from build123d import *

# Parameters (mm, degrees)
F0_R     = 2.4
F1_DEPTH = 3.7
F0_R_2   = 40
F2_DEPTH = 2
F3_R     = 0.5


with BuildPart() as f1:
    # F0 (on Top) → F1 (new body)
    with BuildSketch(Plane.XY):
        with Locations((8, 16)):
            Circle(F0_R)
        with Locations((16, 8)):
            Circle(F0_R)
        with Locations((24, 8)):
            Circle(F0_R)
        with Locations((16, 16)):
            Circle(F0_R)
        with Locations((24, 16)):
            Circle(F0_R)
        with Locations((32, 0)):
            Circle(F0_R)
        with Locations((32, 8)):
            Circle(F0_R)
        with Locations((32, 16)):
            Circle(F0_R)
        with Locations((32, 24)):
            Circle(F0_R)
        with Locations((24, 24)):
            Circle(F0_R)
        with Locations((16, 24)):
            Circle(F0_R)
        with Locations((8, 24)):
            Circle(F0_R)
        with Locations((0, 32)):
            Circle(F0_R)
        with Locations((8, 32)):
            Circle(F0_R)
        with Locations((16, 32)):
            Circle(F0_R)
        with Locations((24, 32)):
            Circle(F0_R)
        with Locations((32, 32)):
            Circle(F0_R)
        with Locations((32, 40)):
            Circle(F0_R)
        with Locations((24, 40)):
            Circle(F0_R)
        with Locations((16, 40)):
            Circle(F0_R)
        with Locations((8, 40)):
            Circle(F0_R)
        with Locations((0, 40)):
            Circle(F0_R)
        with Locations((8, 48)):
            Circle(F0_R)
        with Locations((16, 48)):
            Circle(F0_R)
        with Locations((32, 48)):
            Circle(F0_R)
        with Locations((32, 56)):
            Circle(F0_R)
        with Locations((24, 56)):
            Circle(F0_R)
        with Locations((16, 56)):
            Circle(F0_R)
        with Locations((8, 56)):
            Circle(F0_R)
        with Locations((24, 48)):
            Circle(F0_R)
        with Locations((16, 64)):
            Circle(F0_R)
        with Locations((24, 64)):
            Circle(F0_R)
        with Locations((32, 64)):
            Circle(F0_R)
        with Locations((32, 72)):
            Circle(F0_R)
        with Locations((40, 72)):
            Circle(F0_R)
        with Locations((40, 64)):
            Circle(F0_R)
        with Locations((40, 56)):
            Circle(F0_R)
        with Locations((40, 48)):
            Circle(F0_R)
        with Locations((40, 40)):
            Circle(F0_R)
        with Locations((40, 32)):
            Circle(F0_R)
        with Locations((40, 24)):
            Circle(F0_R)
        with Locations((40, 16)):
            Circle(F0_R)
        with Locations((40, 8)):
            Circle(F0_R)
        with Locations((40, 0)):
            Circle(F0_R)
        with Locations((48, 8)):
            Circle(F0_R)
        with Locations((48, 16)):
            Circle(F0_R)
        with Locations((48, 24)):
            Circle(F0_R)
        with Locations((48, 32)):
            Circle(F0_R)
        with Locations((48, 40)):
            Circle(F0_R)
        with Locations((48, 48)):
            Circle(F0_R)
        with Locations((48, 56)):
            Circle(F0_R)
        with Locations((48, 64)):
            Circle(F0_R)
        with Locations((56, 64)):
            Circle(F0_R)
        with Locations((56, 56)):
            Circle(F0_R)
        with Locations((56, 48)):
            Circle(F0_R)
        with Locations((56, 40)):
            Circle(F0_R)
        with Locations((56, 32)):
            Circle(F0_R)
        with Locations((56, 24)):
            Circle(F0_R)
        with Locations((56, 16)):
            Circle(F0_R)
        with Locations((56, 8)):
            Circle(F0_R)
        with Locations((64, 16)):
            Circle(F0_R)
        with Locations((64, 24)):
            Circle(F0_R)
        with Locations((64, 32)):
            Circle(F0_R)
        with Locations((64, 40)):
            Circle(F0_R)
        with Locations((64, 48)):
            Circle(F0_R)
        with Locations((64, 56)):
            Circle(F0_R)
        with Locations((72, 40)):
            Circle(F0_R)
        with Locations((72, 32)):
            Circle(F0_R)
    extrude(amount=F1_DEPTH)

    # F0 (on Top) → F2 (join)
    with BuildSketch(Plane.XY):
        with Locations((36, 36)):
            Circle(F0_R_2)
        with Locations((32, 0)):
            Circle(F0_R, mode=Mode.SUBTRACT)
        with Locations((16, 8)):
            Circle(F0_R, mode=Mode.SUBTRACT)
        with Locations((24, 8)):
            Circle(F0_R, mode=Mode.SUBTRACT)
        with Locations((32, 8)):
            Circle(F0_R, mode=Mode.SUBTRACT)
        with Locations((8, 16)):
            Circle(F0_R, mode=Mode.SUBTRACT)
        with Locations((8, 24)):
            Circle(F0_R, mode=Mode.SUBTRACT)
        with Locations((0, 32)):
            Circle(F0_R, mode=Mode.SUBTRACT)
        with Locations((8, 32)):
            Circle(F0_R, mode=Mode.SUBTRACT)
        with Locations((16, 16)):
            Circle(F0_R, mode=Mode.SUBTRACT)
        with Locations((24, 16)):
            Circle(F0_R, mode=Mode.SUBTRACT)
        with Locations((16, 24)):
            Circle(F0_R, mode=Mode.SUBTRACT)
        with Locations((24, 24)):
            Circle(F0_R, mode=Mode.SUBTRACT)
        with Locations((32, 16)):
            Circle(F0_R, mode=Mode.SUBTRACT)
        with Locations((32, 24)):
            Circle(F0_R, mode=Mode.SUBTRACT)
        with Locations((16, 32)):
            Circle(F0_R, mode=Mode.SUBTRACT)
        with Locations((24, 32)):
            Circle(F0_R, mode=Mode.SUBTRACT)
        with Locations((32, 32)):
            Circle(F0_R, mode=Mode.SUBTRACT)
        with Locations((40, 0)):
            Circle(F0_R, mode=Mode.SUBTRACT)
        with Locations((40, 8)):
            Circle(F0_R, mode=Mode.SUBTRACT)
        with Locations((48, 8)):
            Circle(F0_R, mode=Mode.SUBTRACT)
        with Locations((56, 8)):
            Circle(F0_R, mode=Mode.SUBTRACT)
        with Locations((40, 16)):
            Circle(F0_R, mode=Mode.SUBTRACT)
        with Locations((40, 24)):
            Circle(F0_R, mode=Mode.SUBTRACT)
        with Locations((48, 16)):
            Circle(F0_R, mode=Mode.SUBTRACT)
        with Locations((48, 24)):
            Circle(F0_R, mode=Mode.SUBTRACT)
        with Locations((40, 32)):
            Circle(F0_R, mode=Mode.SUBTRACT)
        with Locations((48, 32)):
            Circle(F0_R, mode=Mode.SUBTRACT)
        with Locations((56, 16)):
            Circle(F0_R, mode=Mode.SUBTRACT)
        with Locations((64, 16)):
            Circle(F0_R, mode=Mode.SUBTRACT)
        with Locations((56, 24)):
            Circle(F0_R, mode=Mode.SUBTRACT)
        with Locations((64, 24)):
            Circle(F0_R, mode=Mode.SUBTRACT)
        with Locations((56, 32)):
            Circle(F0_R, mode=Mode.SUBTRACT)
        with Locations((64, 32)):
            Circle(F0_R, mode=Mode.SUBTRACT)
        with Locations((72, 32)):
            Circle(F0_R, mode=Mode.SUBTRACT)
        with Locations((0, 40)):
            Circle(F0_R, mode=Mode.SUBTRACT)
        with Locations((8, 40)):
            Circle(F0_R, mode=Mode.SUBTRACT)
        with Locations((8, 48)):
            Circle(F0_R, mode=Mode.SUBTRACT)
        with Locations((16, 40)):
            Circle(F0_R, mode=Mode.SUBTRACT)
        with Locations((24, 40)):
            Circle(F0_R, mode=Mode.SUBTRACT)
        with Locations((32, 40)):
            Circle(F0_R, mode=Mode.SUBTRACT)
        with Locations((16, 48)):
            Circle(F0_R, mode=Mode.SUBTRACT)
        with Locations((24, 48)):
            Circle(F0_R, mode=Mode.SUBTRACT)
        with Locations((32, 48)):
            Circle(F0_R, mode=Mode.SUBTRACT)
        with Locations((8, 56)):
            Circle(F0_R, mode=Mode.SUBTRACT)
        with Locations((16, 56)):
            Circle(F0_R, mode=Mode.SUBTRACT)
        with Locations((24, 56)):
            Circle(F0_R, mode=Mode.SUBTRACT)
        with Locations((16, 64)):
            Circle(F0_R, mode=Mode.SUBTRACT)
        with Locations((24, 64)):
            Circle(F0_R, mode=Mode.SUBTRACT)
        with Locations((32, 56)):
            Circle(F0_R, mode=Mode.SUBTRACT)
        with Locations((32, 64)):
            Circle(F0_R, mode=Mode.SUBTRACT)
        with Locations((32, 72)):
            Circle(F0_R, mode=Mode.SUBTRACT)
        Polygon((37, 33.5), (35, 33.5), (35, 35), (33.5, 35), (33.5, 37), (35, 37), (35, 38.5), (37, 38.5), (37, 37), (38.5, 37), (38.5, 35), (37, 35), align=None, mode=Mode.SUBTRACT)
        with Locations((40, 40)):
            Circle(F0_R, mode=Mode.SUBTRACT)
        with Locations((48, 40)):
            Circle(F0_R, mode=Mode.SUBTRACT)
        with Locations((40, 48)):
            Circle(F0_R, mode=Mode.SUBTRACT)
        with Locations((48, 48)):
            Circle(F0_R, mode=Mode.SUBTRACT)
        with Locations((56, 40)):
            Circle(F0_R, mode=Mode.SUBTRACT)
        with Locations((64, 40)):
            Circle(F0_R, mode=Mode.SUBTRACT)
        with Locations((72, 40)):
            Circle(F0_R, mode=Mode.SUBTRACT)
        with Locations((56, 48)):
            Circle(F0_R, mode=Mode.SUBTRACT)
        with Locations((64, 48)):
            Circle(F0_R, mode=Mode.SUBTRACT)
        with Locations((40, 56)):
            Circle(F0_R, mode=Mode.SUBTRACT)
        with Locations((40, 64)):
            Circle(F0_R, mode=Mode.SUBTRACT)
        with Locations((48, 56)):
            Circle(F0_R, mode=Mode.SUBTRACT)
        with Locations((48, 64)):
            Circle(F0_R, mode=Mode.SUBTRACT)
        with Locations((40, 72)):
            Circle(F0_R, mode=Mode.SUBTRACT)
        with Locations((56, 56)):
            Circle(F0_R, mode=Mode.SUBTRACT)
        with Locations((64, 56)):
            Circle(F0_R, mode=Mode.SUBTRACT)
        with Locations((56, 64)):
            Circle(F0_R, mode=Mode.SUBTRACT)
    extrude(amount=F2_DEPTH)

    # F3
    f3_edges = [f1.edges().sort_by_distance(p)[0] for p in [
        (37, 35, 1),
        (37, 37, 1),
        (35, 37, 1),
        (35, 35, 1),
    ]]
    fillet(f3_edges, radius=F3_R)


solid = f1.part
Source: CAD feature listing. Evaluate the final solid. Frame: model axes, mm. A direction names the side the tool comes from. Give positions to 0.01 mm unless a question says otherwise; leave off trailing zeros. Write each loop counter-clockwise with the first axis right and the second up, starting at its lowest first coordinate (ties: lowest second). Pieces come first, ordered by that corner, then holes. Notation, with made-up numbers: M 22.25,33.25 L 78.25,33.25 A30 ccw 78.25,63.25 Z; hole C -24,11 d3. An arc over 180 degrees is marked long. Return JSON: item names as keys, results as strings. Group by question number.
1) First-contact query: pin 1 Ø1 at (x, z) = (36, 1) entering from +Y; pin 2 Ø0.5 at (y, z) = (38, 1) entering from +X; pin 3 Ø1.1 at (y, z) = (34, 1) entering from -X; pin 4 Ø10 at (x, y) = (51.5, 59) entering from -Z. Flat tips, straight axial feed; report the tip coordinate or a pass-through.
2) Ray query, L1, parallel to Z at x = 69.5, y = 41; L2, parallel to X at y = 9, z = 2.3; L3, parallel to Y at x = 18.5, z = 1. Return the intervals inside material, ascending.
3) Draft query along X for faces 1 (the face through (34.29, 16.72, 2.84)), 2 (the face through (64, 56, 3.7)), 3 (the face through (57.11, 37.87, 2.84)). Return one class per face: released by +X, released by -X, zero draft, split by the parting line, or undercut.
4) Set-up query: faces 4 (the face through (36, 33.5, 1)), 5 (the face through (7.48, 29.657, 2.838)), 6 (the face through (16, 24, 3.7)). Return all of +Z, -Z, +X, -X, +Y, -Y with unobstructed straight access to the full face (end or side cutting, diameter ignored); none if empty.
5) Cut plane A-A, the plane x = 36. Output: boundary loops of the cut face in (y, z), then the cut area to 3 significant figures.
6) Cut plane B-B, the plane z = 0.65. Output: boundary loops of the cut face in (x, y), then the cut area to 3 significant figures.
7) Cut plane D-D, the plane y = 72. Output: boundary loops of the cut face in (x, z).
Data:
{
 "1": {"pin 1": "stops at y = 76", "pin 2": "stops at x = 75.96", "pin 3": "stops at x = -3.97", "pin 4": "stops at z = 0"},
 "2": {"L1": "z = 0 to 2", "L2": "x = 13.82 to 18.18, 21.82 to 26.18, 29.82 to 34.18, 37.82 to 42.18, 45.82 to 50.18, 53.82 to 58.18", "L3": "y = 0.03 to 71.97"},
 "3": {"face 1": "undercut", "face 2": "zero draft", "face 3": "undercut"},
 "4": {"face 4": "+Z, -Z", "face 5": "+Z", "face 6": "+Z, +X, -X, +Y, -Y"},
 "5": {"outline": "M -4,0 L 33.5,0 L 33.5,2 L -4,2 Z; M 38.5,0 L 76,0 L 76,2 L 38.5,2 Z", "area": "150 mm²"},
 "6": {"outline": "C 36,36 d80; hole M 33.5,35 L 34.5,35 A0.5 cw 35,34.5 L 35,33.5 L 37,33.5 L 37,34.5 A0.5 cw 37.5,35 L 38.5,35 L 38.5,37 L 37.5,37 A0.5 cw 37,37.5 L 37,38.5 L 35,38.5 L 35,37.5 A0.5 cw 34.5,37 L 33.5,37 Z", "area": "5,010 mm²"},
 "7": {"outline": "M 18.56,0 L 53.44,0 L 53.44,2 L 42.4,2 L 42.4,3.7 L 37.6,3.7 L 37.6,2 L 34.4,2 L 34.4,3.7 L 29.6,3.7 L 29.6,2 L 18.56,2 Z"}
}
